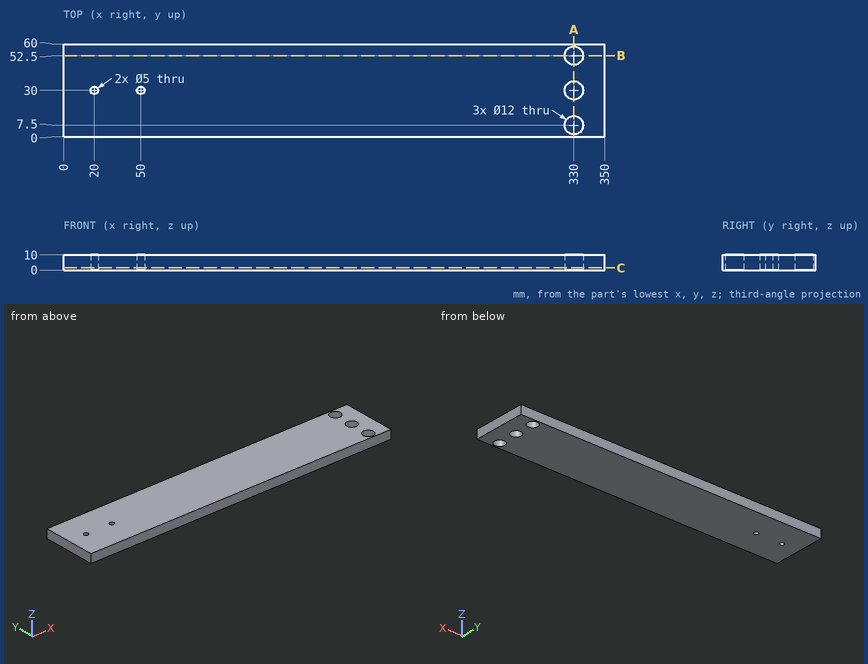
Could you check a few things on this drawing? It's one solid part, dimensions in mm from its lowest x, y, z. Give positions to 0.01 mm unless a question says otherwise; leave off trailing zeros. Write each loop counter-clockwise with the first axis right and the second up, starting at its lowest first coordinate (ties: lowest second). Pieces come first, ordered by that corner, then holes. Notation, with made-up numbers: (52.5, 58) -> (103.5, 58) arc R18 cw to (103.5, 89) -> close; hole circle Ø11 at (-12, 14.5). An arc over 180 degrees is marked (long way). Answer as CSV lines item,"result". Start each with the question number.
(1) Please list where these lines run through material, in increasing order: line 1 (Y direction, x = 330, z = 7.75); line 2 (Y direction, x = 20, z = 3.5); line 3 (X direction, y = 53, z = 2.25).
(2) If we section it at B-B, the plane y = 52.5: Write out the boundary of the cut face in (x, z).
(3) If we section it at C-C, the plane z = 1.5: Write out the boundary of the cut face in (x, y).
(4) If we section it at A-A, the plane x = 330: Write out the boundary of the cut face in (y, z).
(5) I'm going to push a flat-ended pin straight in: pin 1 Ø3 at (x, y) = (20, 30) entering from +Z. Where does the tip first touch, or does it pass through?
Answer list:
1,line 1,"0 to 1.5, 13.5 to 24, 36 to 46.5, 58.5 to 60"
1,line 2,"0 to 27.5, 32.5 to 60"
1,line 3,"0 to 324.02, 335.98 to 350"
2,outline,"(0, 0) -> (324, 0) -> (324, 10) -> (0, 10) -> close; (336, 0) -> (350, 0) -> (350, 10) -> (336, 10) -> close"
3,outline,"(0, 0) -> (350, 0) -> (350, 60) -> (0, 60) -> close; hole circle Ø5 at (20, 30); hole circle Ø5 at (50, 30); hole circle Ø12 at (330, 7.5); hole circle Ø12 at (330, 30); hole circle Ø12 at (330, 52.5)"
4,outline,"(0, 0) -> (1.5, 0) -> (1.5, 10) -> (0, 10) -> close; (13.5, 0) -> (24, 0) -> (24, 10) -> (13.5, 10) -> close; (36, 0) -> (46.5, 0) -> (46.5, 10) -> (36, 10) -> close; (58.5, 0) -> (60, 0) -> (60, 10) -> (58.5, 10) -> close"
5,pin 1,"through"
